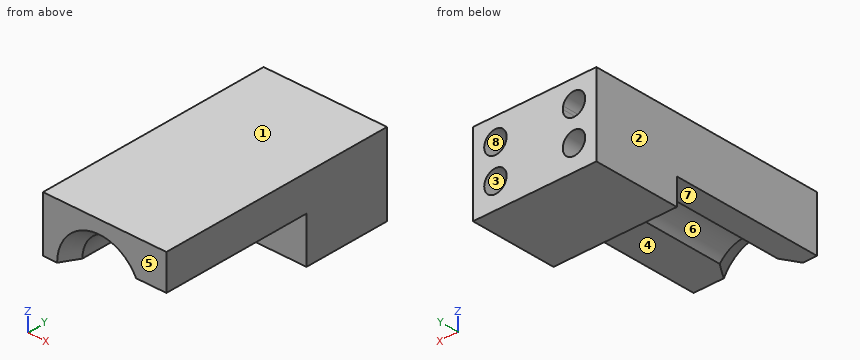
from build123d import *

# Parameters (mm, degrees)
F0_R     = 1.62
F0_R_2   = 2
F1_DEPTH = 15.5
F3_DEPTH = 27
F4_D     = 4
F4_DEPTH = 8
F4_TIP   = 1.2017212381
F5_DEPTH = 6
F6_SIZE2 = 1.7320508076
F6_SIZE  = 3


# Not quite as in the source:
# - ends of sketch curves that miss each other by under 0.0002 mm in the source are joined


with BuildPart() as f1:
    # F0 (on Front) → F1 (new body)
    with BuildSketch(Plane.XZ):
        with BuildLine():
            Line((-81.938941, 0.95), (-79.867763328, 0.95))
            ThreePointArc((-79.867763328, 0.95), (-84.599863166, 4.7050416476), (-90.5653650686, 3.7532564808))
            ThreePointArc((-90.5653650686, 3.7532564808), (-90.517166249, 3.503677095), (-90.501013, 3.25))
            ThreePointArc((-90.501013, 3.25), (-91.2509614327, 1.6887917887), (-92.9383840791, 1.2984092286))
            ThreePointArc((-92.9383840791, 1.2984092286), (-93.5417590804, 0.0341622689), (-93.899505073, -1.3202378094))
            ThreePointArc((-93.899505073, -1.3202378094), (-93.0082544766, -0.8153925244), (-91.9839548989, -0.8179930331))
            ThreePointArc((-91.9839548989, -0.8179930331), (-87.4977327048, 3.112954161), (-81.938941, 0.95))
        make_face()
        with BuildLine():
            ThreePointArc((-90.5653650686, 3.7532564808), (-84.599863166, 4.7050416476), (-79.867763328, 0.9499998269))
            Line((-79.867763328, 0.9499998269), (-74.501013, 0.95))
            Line((-74.501013, 0.95), (-74.501013, 7.25))
            Line((-74.501013, 7.25), (-96.501013, 7.25))
            Line((-96.501013, 7.25), (-96.501013, -2.55))
            Line((-96.501013, -2.55), (-94.4909878742, -2.55))
            ThreePointArc((-94.4909878742, -2.55), (-94.3033741804, -1.8831123628), (-93.899505073, -1.3202378094))
            ThreePointArc((-93.899505073, -1.3202378094), (-93.5417590804, 0.0341622689), (-92.9383840791, 1.2984092286))
            ThreePointArc((-92.9383840791, 1.2984092286), (-93.9389897521, 4.6400441937), (-90.5653650686, 3.7532564808))
        make_face()
        with Locations((-78.501013, 3.25)):
            Circle(F0_R, mode=Mode.SUBTRACT)
        with BuildLine():
            Line((-74.501013, 0.95), (-79.867763328, 0.95))
            Line((-79.867763328, 0.95), (-81.938941, 0.95))
            ThreePointArc((-81.9389410644, 0.9499999506), (-87.4977327048, 3.112954161), (-91.9839548989, -0.8179930331))
            ThreePointArc((-91.9839548989, -0.8179930331), (-92.0381964068, -1.0001290636), (-92.086389397, -1.1839580887))
            ThreePointArc((-92.086389397, -1.1839580887), (-91.2172509043, -1.7618932843), (-90.881013, -2.75))
            ThreePointArc((-90.881013, -2.75), (-92.6012048017, -4.3668987609), (-94.1086199171, -2.55))
            Line((-94.1086199171, -2.55), (-94.4909878742, -2.55))
            Line((-94.4909878742, -2.55), (-96.501013, -2.55))
            Line((-96.501013, -2.55), (-96.501013, -7.25))
            Line((-96.501013, -7.25), (-74.501013, -7.25))
            Line((-74.501013, -7.25), (-74.501013, 0.95))
        make_face()
        with Locations((-78.501013, -2.75)):
            Circle(F0_R_2, mode=Mode.SUBTRACT)
        with BuildLine():
            ThreePointArc((-92.9383840791, 1.2984092286), (-91.8934258204, 2.6626657264), (-90.5653650686, 3.7532564808))
            ThreePointArc((-90.5653650686, 3.7532564808), (-93.9389897521, 4.6400441937), (-92.9383840791, 1.2984092286))
        make_face()
        with Locations((-78.501013, -2.75)):
            Circle(F0_R_2)
        with BuildLine():
            ThreePointArc((-90.501013, 3.25), (-90.517166249, 3.503677095), (-90.5653650686, 3.7532564808))
            ThreePointArc((-90.5653650686, 3.7532564808), (-91.8934258204, 2.6626657264), (-92.9383840791, 1.2984092286))
            ThreePointArc((-92.9383840791, 1.2984092286), (-91.2509614327, 1.6887917887), (-90.501013, 3.25))
        make_face()
        with Locations((-78.501013, 3.25)):
            Circle(F0_R)
        with BuildLine():
            ThreePointArc((-93.9879149105, -2.1069426863), (-93.9540972375, -1.7124229299), (-93.899505073, -1.3202378094))
            ThreePointArc((-93.899505073, -1.3202378094), (-94.3033741804, -1.8831123628), (-94.4909878742, -2.55))
            Line((-94.4909878742, -2.55), (-94.1086199171, -2.55))
            ThreePointArc((-94.1086199171, -2.55), (-94.0640456826, -2.324172766), (-93.9879149105, -2.1069426863))
        make_face()
        with BuildLine():
            ThreePointArc((-92.086389397, -1.1839580887), (-92.0381964068, -1.0001290636), (-91.9839548989, -0.8179930331))
            ThreePointArc((-91.9839548989, -0.8179930331), (-93.0082544766, -0.8153925244), (-93.899505073, -1.3202378094))
            ThreePointArc((-93.899505073, -1.3202378094), (-93.9540972375, -1.7124229299), (-93.9879149105, -2.1069426863))
            ThreePointArc((-93.9879149105, -2.1069426863), (-93.2084169398, -1.29261204), (-92.086389397, -1.1839580887))
        make_face()
        with BuildLine():
            ThreePointArc((-90.881013, -2.75), (-91.2172509043, -1.7618932843), (-92.086389397, -1.1839580887))
            ThreePointArc((-92.086389397, -1.1839580887), (-92.2097087478, -1.8620371678), (-92.251013, -2.55))
            Line((-92.251013, -2.55), (-94.001013, -2.55))
            Line((-94.001013, -2.55), (-94.1086199171, -2.55))
            ThreePointArc((-94.1086199171, -2.55), (-92.6012048017, -4.3668987609), (-90.881013, -2.75))
        make_face()
        with BuildLine():
            ThreePointArc((-92.251013, -2.55), (-92.2097087478, -1.8620371678), (-92.086389397, -1.1839580887))
            ThreePointArc((-92.086389397, -1.1839580887), (-93.2084169398, -1.29261204), (-93.9879149105, -2.1069426863))
            ThreePointArc((-93.9879149105, -2.1069426863), (-93.9977377625, -2.3283745597), (-94.001013, -2.55))
            Line((-94.001013, -2.55), (-92.251013, -2.55))
        make_face()
        with BuildLine():
            ThreePointArc((-94.001013, -2.55), (-93.9977377625, -2.3283745597), (-93.9879149105, -2.1069426863))
            ThreePointArc((-93.9879149105, -2.1069426863), (-94.0640456826, -2.324172766), (-94.1086199171, -2.55))
            Line((-94.1086199171, -2.55), (-94.001013, -2.55))
        make_face()
    extrude(amount=F1_DEPTH)

    # F2 (on face) → F3 (join)
    with BuildSketch(Plane.XZ.offset(15.5)):
        with BuildLine():
            Line((-81.938941, 0.95), (-74.501013, 0.95))
            Line((-74.501013, 0.95), (-74.501013, 7.25))
            Line((-74.501013, 7.25), (-96.501013, 7.25))
            Line((-96.501013, 7.25), (-96.501013, -2.55))
            Line((-96.501013, -2.55), (-92.251013, -2.55))
            ThreePointArc((-92.251013, -2.55), (-88.3490641857, 2.8949248677), (-81.9389410644, 0.9499999506))
        make_face()
    extrude(amount=F3_DEPTH)

    # F4
    with Locations(Plane(origin=(0, 0, 0), x_dir=(1, 0, 0), z_dir=(0, 1, 0))):
        with Locations((-92.501013, 2.75), (-78.501013, -3.25)):
            Hole(F4_D / 2, depth=F4_DEPTH)
            with Locations((0, 0, -(F4_DEPTH + F4_TIP / 2))):  # 118° drill point
                Cone(0, F4_D / 2, F4_TIP, mode=Mode.SUBTRACT)

    # F0 (on Front) → F5 (cut)
    with BuildSketch(Plane.XZ):
        with BuildLine():
            ThreePointArc((-92.9383840791, 1.2984092286), (-91.8934258204, 2.6626657264), (-90.5653650686, 3.7532564808))
            ThreePointArc((-90.5653650686, 3.7532564808), (-93.9389897521, 4.6400441937), (-92.9383840791, 1.2984092286))
        make_face()
        with BuildLine():
            ThreePointArc((-90.501013, 3.25), (-90.517166249, 3.503677095), (-90.5653650686, 3.7532564808))
            ThreePointArc((-90.5653650686, 3.7532564808), (-91.8934258204, 2.6626657264), (-92.9383840791, 1.2984092286))
            ThreePointArc((-92.9383840791, 1.2984092286), (-91.2509614327, 1.6887917887), (-90.501013, 3.25))
        make_face()
        with Locations((-78.501013, -2.75)):
            Circle(F0_R_2)
    extrude(amount=F5_DEPTH, mode=Mode.SUBTRACT)

    # F6
    f6_edges = [f1.edges().sort_by_distance(p)[0] for p in [
        (-88.349064, -42.5, 2.894925),
    ]]
    f6_side = f1.faces().sort_by_distance((-88.349064, -29, 2.894925))[0]
    chamfer(f6_edges, length=F6_SIZE, length2=F6_SIZE2, reference=f6_side)


solid = f1.part
Build history of the part. All positions in model axes, mm. Face numbers are marked on the shaded views. A direction names the side the tool comes from. Round coordinates to 2 decimals unless told otherwise and drop trailing zeros. Write each loop counter-clockwise with the first axis right and the second up, starting at its lowest first coordinate (ties: lowest second). Pieces come first, ordered by that corner, then holes. Notation, with made-up numbers: M 16,87 L 66,87 A20 cw 66,106 Z; hole C -18,78 d3. An arc over 180 degrees is marked long. Use CSV: the item, a comma, the result in double quotes.
1. Wall check: probe 1 along Y at (x, z) = (-83, -1); probe 2 along Z at (x, y) = (-93.75, -2.5); probe 3 along Z at (x, y) = (-93.25, -26). Give the ranges that are in metal, low to high. Write a range as from..to.
Reply:
probe 1,"y = -15.5..0"
probe 2,"z = -7.25..-4.31, -1.19..1.69, 4.81..7.25"
probe 3,"z = -2.55..7.25"
2. Flat gauge pins, fed straight in: pin 1 (2 mm diameter, centred on x = -92.5, y = -37, fed in from -Z); pin 2 (2 mm diameter, centred on x = -78, z = -3.5, fed in from +Y); pin 3 (5 mm diameter, centred on x = -83.5, y = -30.5, fed in from -Z). Where does each tip first touch, or does it go through?
Reply:
pin 1,"stops at z = -2.55"
pin 2,"stops at y = -6"
pin 3,"stops at z = 0.95"
3. Saw through at A-A (y = -27). Give the cut face in (x, z).
Reply:
outline,"M -96.5,-2.55 L -92.25,-2.55 A5.75 cw -81.94,0.95 L -74.5,0.95 L -74.5,7.25 L -96.5,7.25 Z"
4. Saw through at B-B (z = -5.5). Give the cut face in (x, y), plus the area to 3 significant figures.
Reply:
outline,"M -96.5,-15.5 L -74.5,-15.5 L -74.5,0 L -96.5,0 Z"
area,"341 mm²"
5. Two-plate mould, pull along X, no slides. Class the marked faces 1, 2 and 3: +X half, -X half, draft (parallel to the pull), parting line (faces both ways), or undercut.
Reply:
face 1,"draft"
face 2,"-X half"
face 3,"undercut"
6. Tool access for the marked faces 4, 5, 6, 7 and 8: list every direction of +Z, -Z, +X, -X, +Y, -Y with a clear straight run to the whole face (end or side of a thin tool).
Reply:
face 4,"-Z, +X, -Y"
face 5,"+Z, -Z, +X, -X, -Y"
face 6,"-Z, -Y"
face 7,"-Z, +X, -X, -Y"
face 8,"+Y"
